```python
from build123d import *

# Parameters (mm, degrees)
SKETCH3_W           = 92
SKETCH3_H           = 63
SKETCH3_R           = 3
SKETCH3_R_2         = 2.25
SKETCH3_W_2         = 7
SKETCH3_H_2         = 10
BOSS_EXTRUDE3_DEPTH = 25
SKETCH4_W           = 84
SKETCH4_H           = 55
CUT_EXTRUDE1_DEPTH  = 23
SKETCH5_W           = 88
SKETCH5_H           = 59
CUT_EXTRUDE2_DEPTH  = 5
FILLET1_R           = 3
SKETCH6_W           = 15
SKETCH6_H           = 21
CUT_EXTRUDE3_DEPTH  = 5


with BuildPart() as part:
    # Sketch3 → Boss-Extrude3 (new body)
    with BuildSketch(Plane.XY):
        with Locations((46, 31.5)):
            Rectangle(SKETCH3_W, SKETCH3_H)
        with Locations((35, 31.5)):
            Circle(SKETCH3_R, mode=Mode.SUBTRACT)
        with Locations((57, 31.5)):
            Circle(SKETCH3_R, mode=Mode.SUBTRACT)
        with Locations((77, 31.5)):
            Circle(SKETCH3_R, mode=Mode.SUBTRACT)
        with Locations((82, 53)):
            Circle(SKETCH3_R_2, mode=Mode.SUBTRACT)
        with Locations((82, 10)):
            Circle(SKETCH3_R_2, mode=Mode.SUBTRACT)
        with Locations((10.5, 10)):
            Circle(SKETCH3_R_2, mode=Mode.SUBTRACT)
        with Locations((10.5, 53)):
            Circle(SKETCH3_R_2, mode=Mode.SUBTRACT)
        with Locations((71.5, 15.5)):
            Rectangle(SKETCH3_W_2, SKETCH3_H_2, mode=Mode.SUBTRACT)
        with Locations((54, 15.5)):
            Rectangle(SKETCH3_W_2, SKETCH3_H_2, mode=Mode.SUBTRACT)
        with Locations((36, 15.5)):
            Rectangle(SKETCH3_W_2, SKETCH3_H_2, mode=Mode.SUBTRACT)
    extrude(amount=BOSS_EXTRUDE3_DEPTH)

    # Sketch4 → Cut-Extrude1 (cut)
    with BuildSketch(Plane.XY.offset(25)):
        with Locations((46, 31.5)):
            Rectangle(SKETCH4_W, SKETCH4_H)
    extrude(amount=-CUT_EXTRUDE1_DEPTH, mode=Mode.SUBTRACT)

    # Sketch5 → Cut-Extrude2 (cut)
    with BuildSketch(Plane.XY.offset(25)):
        with Locations((46, 31.5)):
            Rectangle(SKETCH5_W, SKETCH5_H)
    extrude(amount=-CUT_EXTRUDE2_DEPTH, mode=Mode.SUBTRACT)

    # Fillet1
    fillet1_edges = [part.edges().sort_by_distance(p)[0] for p in [
        (0, 31.5, 0),
        (46, 63, 0),
        (92, 31.5, 0),
        (46, 0, 0),
    ]]
    fillet(fillet1_edges, radius=FILLET1_R)

    # Sketch6 → Cut-Extrude3 (cut)
    with BuildSketch(Plane.ZY):
        with Locations((14.5, 28.5)):
            Rectangle(SKETCH6_W, SKETCH6_H)
    extrude(amount=-CUT_EXTRUDE3_DEPTH, mode=Mode.SUBTRACT)


solid = part.part
```
The listing builds one solid part. Answer for the finished solid, in the listing's coordinates (mm). A direction names the side the tool comes from. Give positions to 0.01 mm unless a question says otherwise; leave off trailing zeros. Loops run counter-clockwise (first coordinate to the right, second up) from the corner with the lowest first, then second, coordinate; pieces in that order, holes last. Notation, with made-up numbers: M 23,-14 L 53,-14 A24 cw 53,15 Z; hole C 16.25,-40 d5. An arc over 180 degrees is marked long. One line per item, written item: value.
1. Each of these flat-tipped pins is pushed along its axis until it touches: P1, Ø2, axis at x = 55, z = 1, coming from the -Y side; P2, Ø16.5, axis at x = 48.5, y = 37.5, coming from the +Z side; P3, Ø5, axis at x = 77, y = 31.5, coming from the +Z side; P4, Ø1, axis at x = 72.5, z = 0.5, coming from the -Y side. Where does it stop, or does it pass through?
Found:
P1: y = 0.17
P2: z = 2
P3: through
P4: y = 0.76
2. Section D-D on x = 52 is taken. Determine the outline of the cut face in (y, z).
Found:
outline: M 0,3 A3 ccw 3,0 L 10.5,0 L 10.5,2 L 4,2 L 4,20 L 2,20 L 2,25 L 0,25 Z; M 20.5,0 L 60,0 A3 ccw 63,3 L 63,25 L 61,25 L 61,20 L 59,20 L 59,2 L 20.5,2 Z
3. Section B-B on y = 25 is taken. Determine the outline of the cut face in (x, z).
Found:
outline: M 0,3 A3 ccw 3,0 L 89,0 A3 ccw 92,3 L 92,25 L 90,25 L 90,20 L 88,20 L 88,2 L 4,2 L 4,7 L 0,7 Z; M 0,22 L 2,22 L 2,25 L 0,25 Z
4. Section A-A on x = 82 is taken. Determine the outline of the cut face in (y, z).
Found:
outline: M 0,3 A3 ccw 3,0 L 7.75,0 L 7.75,2 L 4,2 L 4,20 L 2,20 L 2,25 L 0,25 Z; M 12.25,0 L 50.75,0 L 50.75,2 L 12.25,2 Z; M 55.25,0 L 60,0 A3 ccw 63,3 L 63,25 L 61,25 L 61,20 L 59,20 L 59,2 L 55.25,2 Z
5. Find the intervals of material crossed by probe 1 along Y at (x, z) = (57, 19.25); probe 2 along X at (y, z) = (13, 2.75); probe 3 along Y at (x, z) = (72, 23.5), in increasing order.
Found:
probe 1: 0 to 4, 59 to 63
probe 2: 0.01 to 4, 88 to 91.99
probe 3: 0 to 2, 61 to 63
6. For a pull along X with two mould halves and no side action, classify faces 1 (the face through (10.21, 55.23, 0.99)), 2 (the face through (2, 18, 14)), 3 (the face through (92, 31, 14)) as pulls with the +X half, pulls with the -X half, needs draft (parallel to the pull), parting line crosses it, or undercut.
Found:
face 1: undercut
face 2: needs draft
face 3: pulls with the +X half
7. Section C-C on y = 53 is taken. Determine the outline of the cut face in (x, z).
Found:
outline: M 0,3 A3 ccw 3,0 L 8.25,0 L 8.25,2 L 4,2 L 4,20 L 2,20 L 2,25 L 0,25 Z; M 12.75,0 L 79.75,0 L 79.75,2 L 12.75,2 Z; M 84.25,0 L 89,0 A3 ccw 92,3 L 92,25 L 90,25 L 90,20 L 88,20 L 88,2 L 84.25,2 Z
8. For faces 4 (the face through (45, 32, 0)), 5 (the face through (39.5, 15, 1)), 6 (the face through (45, 4, 11)), 7 (the face through (1, 28, 22)), 8 (the face through (91.1, 31.94, 0.86)), determine the directions among +Z, -Z, +X, -X, +Y, -Y from which every point of the face is accessible in a straight line to the end or side of a thin tool.
Found:
face 4: -Z, +X, -X, +Y, -Y
face 5: +Z, -Z
face 6: +Z
face 7: -X
face 8: -Z, +X, +Y, -Y
